Input: dimensioned drawing with shaded views. Units: mm. Origin: part minimum x, y, z. Round coordinates to 2 decimals unless told otherwise and drop trailing zeros. Order: outer loops, then holes, each group sorted by start corner. A loop starts at its lowest first (then second) coordinate and runs counter-clockwise, first axis right, second up. Notation, with made-up numbers: M -9.75,-31 L 41.25,-31 A20 cw 41.25,-8 Z; hole C 15,-30 d11. An arc over 180 degrees is marked long. Use CSV: the item, a comma, the result in double quotes. Start each with the question number.
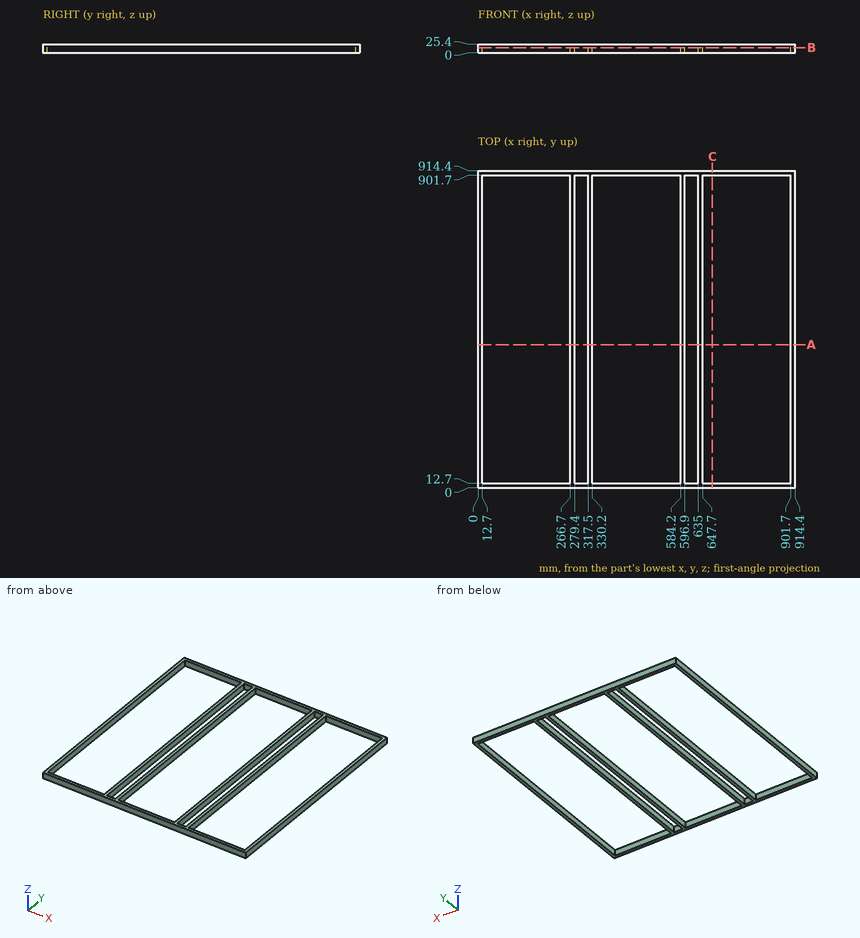
(1) Line query: line 1 along X through (y, z) = (259.5, 21); line 2 along Y through (x, z) = (122.5, 21). Output: solid intervals per line, ascending.
(2) Section A-A on y = 413. Return loops of the section in (x, z), plus the area to 3 significant figures.
(3) Section C-C on x = 676. Return loops of the section in (y, z).
(4) Section B-B on z = 15. Return loops of the section in (x, y).
Results below:
1,line 1,"x = 0 to 12.7, 266.7 to 279.4, 317.5 to 330.2, 584.2 to 596.9, 635 to 647.7, 901.7 to 914.4"
1,line 2,"y = 0 to 12.7, 901.7 to 914.4"
2,outline,"M 0,0 L 12.7,0 L 12.7,25.4 L 0,25.4 Z; M 266.7,0 L 279.4,0 L 279.4,25.4 L 266.7,25.4 Z; M 317.5,0 L 330.2,0 L 330.2,25.4 L 317.5,25.4 Z; M 584.2,0 L 596.9,0 L 596.9,25.4 L 584.2,25.4 Z; M 635,0 L 647.7,0 L 647.7,25.4 L 635,25.4 Z; M 901.7,0 L 914.4,0 L 914.4,25.4 L 901.7,25.4 Z"
2,area,"1,940 mm2"
3,outline,"M 0,0 L 12.7,0 L 12.7,25.4 L 0,25.4 Z; M 901.7,0 L 914.4,0 L 914.4,25.4 L 901.7,25.4 Z"
4,outline,"M 0,0 L 914.4,0 L 914.4,914.4 L 0,914.4 Z; hole M 12.7,12.7 L 266.7,12.7 L 266.7,901.7 L 12.7,901.7 Z; hole M 279.4,12.7 L 317.5,12.7 L 317.5,901.7 L 279.4,901.7 Z; hole M 330.2,12.7 L 584.2,12.7 L 584.2,901.7 L 330.2,901.7 Z; hole M 596.9,12.7 L 635,12.7 L 635,901.7 L 596.9,901.7 Z; hole M 647.7,12.7 L 901.7,12.7 L 901.7,901.7 L 647.7,901.7 Z"
